```python
from build123d import *

# Parameters (mm, degrees)
F0_R     = 1.5
F1_DEPTH = 52
F2_R     = 3
F2_R_2   = 1.5
F3_DEPTH = 6
F5_DEPTH = 5
F6_R     = 1


with BuildPart() as f1:
    # F0 (on Top) → F1 (new body)
    with BuildSketch(Plane.XY):
        Circle(F0_R)
    extrude(amount=F1_DEPTH)

    # F2 (on face) → F3 (join)
    with BuildSketch(Plane.XY.offset(52)):
        Circle(F2_R)
        Circle(F2_R_2, mode=Mode.SUBTRACT)
        Circle(F2_R_2)
    extrude(amount=-F3_DEPTH)

    # F4 (on face) → F5 (cut)
    with BuildSketch(Plane.XY.offset(52)):
        Polygon((0.471543, -1.666628), (1.679113, -0.424946), (1.20757, 1.241682), (-0.471543, 1.666628), (-1.679113, 0.424946), (-1.20757, -1.241682), align=None)
    extrude(amount=-F5_DEPTH, mode=Mode.SUBTRACT)

    # F6
    f6_edges = [f1.edges().sort_by_distance(p)[0] for p in [
        (-1.5, 0, 0),
        (-3, 0, 46),
    ]]
    fillet(f6_edges, radius=F6_R)


solid = f1.part
```
Design review of the part built by this model. Coordinates are the model's own, in mm. A direction names the side the tool comes from. Coordinates: 2 decimals unless noted, no trailing zeros. Loops run counter-clockwise (first coordinate to the right, second up) from the corner with the lowest first, then second, coordinate; pieces in that order, holes last. Notation, with made-up numbers: M 45,-7 L 80,-7 A21 ccw 80,5 Z; hole C -39,8 d9. An arc over 180 degrees is marked long. One line per question, with ' | ' between items.
(1) For pin 1 Ø1.5 at (y, z) = (0.5, 41.5) entering from +X; pin 2 Ø1.5 at (x, z) = (-1.5, 37) entering from +Y; pin 3 Ø1.7 at (x, y) = (0.5, 0) entering from +Z, all flat-tipped, find the tip position at first contact; note any pin that passes through.
Filled in:
pin 1: stops at x = 1.5 | pin 2: stops at y = 1.3 | pin 3: stops at z = 47
(2) We need section A-A (z = 8). Give the boundary of the cut face in (x, y).
Filled in:
outline: C 0,0 d3
(3) Draft analysis for pull direction Y (two halves, no side actions). For faces 1 (the face through (1.3, -1.3, 52)), 2 (the face through (-1.5, 0.07, 23.18)), 3 (the face through (0.38, 1.45, 49.54)), state which applies: released by +Y, released by -Y, zero draft, split by the parting line, or undercut.
Filled in:
face 1: zero draft | face 2: split by the parting line | face 3: undercut
(4) Wall thickness on probe 1 along Z at (x, y) = (1.5, 1.5); probe 2 along X at (y, z) = (0, 15); probe 3 along Z at (x, y) = (0.1, 2.5): over which ranges is each line inside the solid? List them lowest first.
Filled in:
probe 1: z = 46.01 to 52 | probe 2: x = -1.5 to 1.5 | probe 3: z = 46.14 to 52
(5) Machinability: for faces 4 (the face through (0, 0, 0)), 5 (the face through (1.447, 0.397, 49.535)), which of the approach directions +Z, -Z, +X, -X, +Y, -Y give a long, thin tool a straight path to every point of the face, cutting with its end or side? Answer none if there is none.
Filled in:
face 4: -Z, +X, -X, +Y, -Y | face 5: +Z
